For this review, use the dimensioned drawing (mm, ordinates from the lowest corner) and the shaded views. A direction names the side the tool comes from. Round coordinates to 2 decimals unless told otherwise and drop trailing zeros. Order: outer loops, then holes, each group sorted by start corner. A loop starts at its lowest first (then second) coordinate and runs counter-clockwise, first axis right, second up. Notation, with made-up numbers: (-39, 59) -> (-1, 59) arc R26 ccw to (-1, 90) -> close; hole circle Ø9 at (87.25, 14). An arc over 180 degrees is marked (long way). Answer in a Markdown table with one row per item.
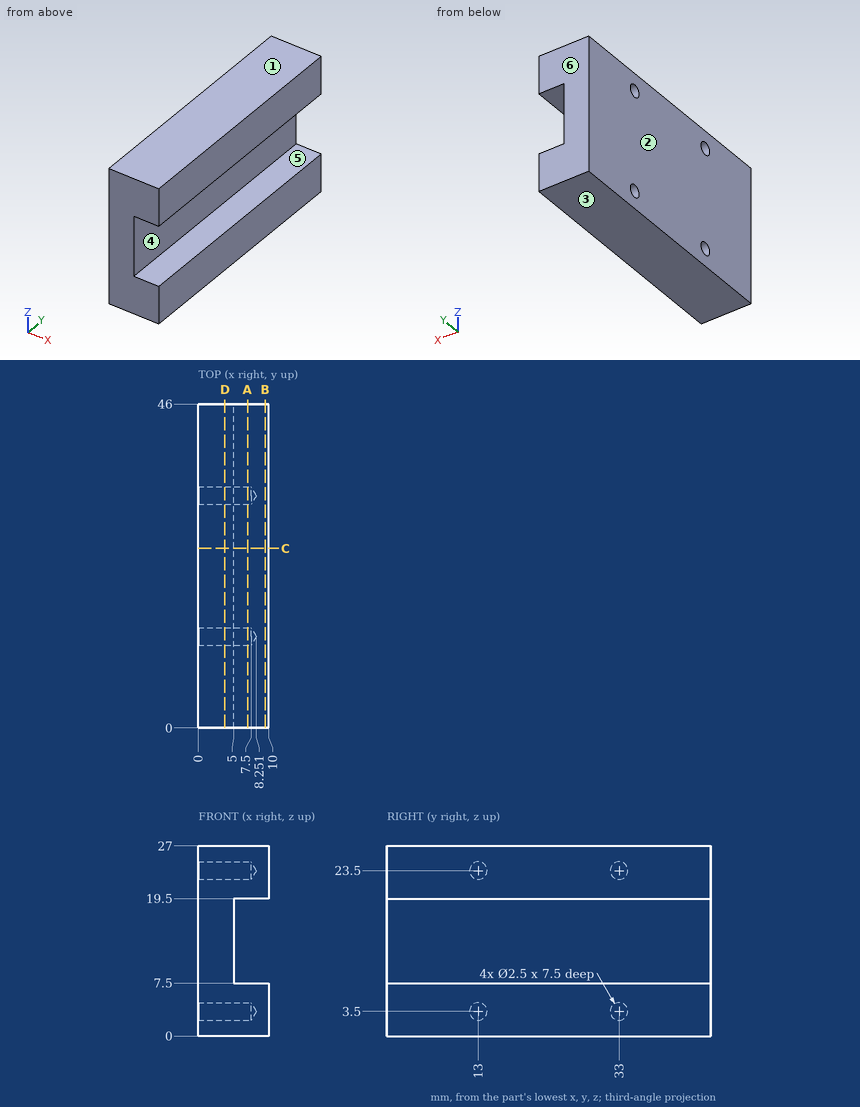
Q1. To check wall thickness, follow probe 1 along Z at (x, y) = (3, 13); probe 2 along Y at (x, z) = (1.75, 3.5); probe 3 along Z at (x, y) = (5.75, 33). State the ranges of each line that lie inside material, in increasing order.
Answer key:
| item | result |
|---|---|
| probe 1 | z = 0 to 2.25, 4.75 to 22.25, 24.75 to 27 |
| probe 2 | y = 0 to 11.75, 14.25 to 31.75, 34.25 to 46 |
| probe 3 | z = 0 to 2.25, 4.75 to 7.5, 19.5 to 22.25, 24.75 to 27 |
Q2. Take a section at C-C, the plane y = 25.5. Write out the cut boundary in (x, z).
Answer key:
| item | result |
|---|---|
| outline | (0, 0) -> (10, 0) -> (10, 7.5) -> (5, 7.5) -> (5, 19.5) -> (10, 19.5) -> (10, 27) -> (0, 27) -> close |
Q3. The part is to be moulded in two halves that separate along Z. For the marked faces 1, 2, 3 and 4, say which applies: +Z half, -Z half, draft (parallel to the pull), parting line (faces both ways), or undercut.
Answer key:
| item | result |
|---|---|
| face 1 | +Z half |
| face 2 | draft |
| face 3 | -Z half |
| face 4 | undercut |
Q4. Take a section at A-A, the plane x = 7. Write out the cut boundary in (y, z).
Answer key:
| item | result |
|---|---|
| outline | (0, 0) -> (46, 0) -> (46, 7.5) -> (0, 7.5) -> close; (0, 19.5) -> (46, 19.5) -> (46, 27) -> (0, 27) -> close; hole circle Ø2.5 at (13, 3.5); hole circle Ø2.5 at (13, 23.5); hole circle Ø2.5 at (33, 3.5); hole circle Ø2.5 at (33, 23.5) |
Q5. Take a section at D-D, the plane x = 3.75. Write out the cut boundary in (y, z), then the cut area to 3 significant figures.
Answer key:
| item | result |
|---|---|
| outline | (0, 0) -> (46, 0) -> (46, 27) -> (0, 27) -> close; hole circle Ø2.5 at (13, 3.5); hole circle Ø2.5 at (13, 23.5); hole circle Ø2.5 at (33, 3.5); hole circle Ø2.5 at (33, 23.5) |
| area | 1,220 mm^2 |
Q6. Take a section at B-B, the plane x = 9.5. Write out the cut boundary in (y, z).
Answer key:
| item | result |
|---|---|
| outline | (0, 0) -> (46, 0) -> (46, 7.5) -> (0, 7.5) -> close; (0, 19.5) -> (46, 19.5) -> (46, 27) -> (0, 27) -> close |
Q7. Tool access review of the marked faces 5 and 6: name each direction out of +Z, -Z, +X, -X, +Y, -Y from which nothing blocks a thin tool from reaching the whole face with its end or side.
Answer key:
| item | result |
|---|---|
| face 5 | +X, +Y, -Y |
| face 6 | +Z, -Z, +X, -X, +Y |
Q8. Clearance check with flat-ended pins moving along their axes: pin 1 Ø2 at (y, z) = (6, 13) entering from +X; pin 2 Ø2 at (y, z) = (13, 23.5) entering from -X. State where each tip first meets the part, or that it passes through.
Answer key:
| item | result |
|---|---|
| pin 1 | stops at x = 5 |
| pin 2 | stops at x = 7.65 |
